from build123d import *

# Parameters (mm, degrees)
BOSS_EXTRUDE1_DEPTH = 355.6
SKETCH3_R           = 1.4224
CUT_EXTRUDE1_DEPTH  = 5.08


with BuildPart() as part:
    # Sketch2 → Boss-Extrude1 (new body)
    with BuildSketch(Plane(origin=(0, 0, 0), x_dir=(1, 0, 0), z_dir=(0, 1, 0))):
        with BuildLine():
            Line((0, 0), (19.05, 0))
            Line((19.05, 0), (19.05, 1.5875))
            ThreePointArc((19.05, 1.5875), (18.585032015, 2.710032015), (17.4625, 3.175))
            Line((17.4625, 3.175), (4.7625, 3.175))
            ThreePointArc((4.7625, 3.175), (3.639967985, 3.639967985), (3.175, 4.7625))
            Line((3.175, 4.7625), (3.175, 17.4625))
            ThreePointArc((3.175, 17.4625), (2.710032015, 18.585032015), (1.5875, 19.05))
            Line((1.5875, 19.05), (0, 19.05))
            Line((0, 19.05), (0, 0))
        make_face()
    extrude(amount=BOSS_EXTRUDE1_DEPTH)

    # Sketch3 → Cut-Extrude1 (cut)
    with BuildSketch(Plane(origin=(0, 0, -3.175), x_dir=(-1, 0, 0), z_dir=(0, 0, -1))):
        with Locations((-11.1125, 7.9375)):
            Circle(SKETCH3_R)
        with Locations((-11.1125, 347.6625)):
            Circle(SKETCH3_R)
        with Locations((-11.1125, 96.8375)):
            Circle(SKETCH3_R)
        with Locations((-11.1125, 177.8)):
            Circle(SKETCH3_R)
        with Locations((-11.1125, 258.7625)):
            Circle(SKETCH3_R)
    extrude(amount=-CUT_EXTRUDE1_DEPTH, mode=Mode.SUBTRACT)


solid = part.part
Here's how the part is built. I have some questions about the finished solid (model axes, mm). A direction names the side the tool comes from. Round coordinates to 2 decimals unless told otherwise and drop trailing zeros. Order: outer loops, then holes, each group sorted by start corner. A loop starts at its lowest first (then second) coordinate and runs counter-clockwise, first axis right, second up. Notation, with made-up numbers: (64.25, 45) -> (75.25, 45) arc R24 ccw to (75.25, 72) -> close; hole circle Ø11 at (-37, 12.25). An arc over 180 degrees is marked (long way). Use CSV: the item, a comma, the result in double quotes.
1. Which directions (+Z, -Z, +X, -X, +Y, -Y) give clear straight access to the entire face, cutting with the end or side of a thin tool? Please do faces 1 (the face through (11, 175, -3.175)), 2 (the face through (9, 175, 0)).
Recorded:
face 1,"-Z, +X, +Y, -Y"
face 2,"+Z, +X, -X, +Y, -Y"
2. I need wall thicknesses on line 1 along Z through (x, y) = (14.25, 146.5) (3 decimals); line 2 along X through (y, z) = (46, -7.75) (3 decimals); line 3 along Z through (x, y) = (2, 216). Which ranges of each line are inside material? Lowest first, please.
Recorded:
line 1,"z = -3.175 to 0"
line 2,"x = 0 to 3.175"
line 3,"z = -19 to 0"
3. I'm going to push flat-ended pins straight in: P1, Ø3.5, axis at x = 11.11, y = 347.66, coming from the -Z side (3 decimals); P2, Ø10, axis at x = 5.5, y = 226.5, coming from the +Z side; P3, Ø1.7, axis at x = 11.11, y = 258.76, coming from the -Z side; P4, Ø10, axis at y = 250.5, z = -9.5, coming from the +X side. Where does each tip first touch, or does it pass through?
Recorded:
P1,"stops at z = -3.175"
P2,"stops at z = 0"
P3,"passes through"
P4,"stops at x = 3.2"
4. I want a section at B-B on z = -8.5. List the corners of the cut face in (x, y) for me (3 decimals), and give its area (3 significant figures).
Recorded:
outline,"(0, 0) -> (3.175, 0) -> (3.175, 355.6) -> (0, 355.6) -> close"
area,"1,130 mm2"
